Autodesk Inventor part; units mm, degrees
ref_plane "YZ Plane" through (0, 0, 0) normal (1, 0, 0) x (0, 1, 0)
ref_plane "XZ Plane" through (0, 0, 0) normal (0, 1, 0) x (-1, 0, 0)
ref_plane "XY Plane" through (0, 0, 0) normal (0, 0, 1) x (1, 0, 0)
sketch "Sketch1" plane through (0, 0, 0) normal (0, 0, 1) x (1, 0, 0)
  circle A0 centre (0, 0) radius 1.621
  dimension "d0" = 3.242
extrude "Extrusion1" add sketch "Sketch1" along normal blind 4.6
sketch "Sketch2" plane through (0, 0, 4.6) normal (0, 0, 1) x (1, 0, 0)
  circle A0 centre (0, 0) radius 2.5
  dimension "d3" = 5
extrude "Extrusion2" add sketch "Sketch2" along normal blind 3
sketch "Sketch3" plane through (0, 0, 7.6) normal (0, 0, 1) x (1, 0, 0)
  line L0 (0.866, 1.5) -> (1.7321, 0)
  line L1 (1.7321, 0) -> (0.866, -1.5)
  line L2 (0.866, -1.5) -> (-0.866, -1.5)
  line L3 (-0.866, -1.5) -> (-1.7321, 0)
  line L4 (-1.7321, 0) -> (-0.866, 1.5)
  line L5 (-0.866, 1.5) -> (0.866, 1.5)
  point P0 (0, 0)
  dimension "d14" = 3
extrude "Extrusion3" cut sketch "Sketch3" against normal blind 2
thread "Thread1"
properties part number "M4 sujecion"
Check sheet for the modelled part. Datum: model origin and axes. Units: mm. A direction names the side the tool comes from. Give positions to 0.01 mm unless a question says otherwise; leave off trailing zeros. Order: outer loops, then holes, each group sorted by start corner. A loop starts at its lowest first (then second) coordinate and runs counter-clockwise, first axis right, second up. Notation, with made-up numbers: M -28,-19 L 4,-19 A11 ccw 4,-1 Z; hole C -23,78.25 d1. An arc over 180 degrees is marked long. Answer as CSV lines item,"result". Start each with the question number.
Item 1: Cross-section at A-A on z = 6.25. Enter the section's corners in (x, y).
Item 2: Mould release check, pull along Y, two halves, no side actions. Record for faces 1 (the face through (-0.54, 2.44, 6.08)), 2 (the face through (0, 0, 0)), 3 (the face through (0, -1.5, 7)): +Y half, -Y half, draft (parallel to the pull), parting line (faces both ways), or undercut.
Item 3: Cross-section at B-B on x = 0. Enter the section's corners in (y, z), plus the area to 3 significant figures.
Item 4: Gauge pin test, flat ends, axial feed: P1, Ø1, axis at x = -1, z = 5, coming from the +Y side; P2, Ø1.5, axis at x = 0.5, y = 0, coming from the +Z side; P3, Ø3, axis at x = -1, z = 1, coming from the +Y side. Record the tip position at first contact, or that the pin passes through.
Item 5: Cross-section at C-C on y = 1.2. Enter the section's corners in (x, z).
Item 6: Cross-section at D-D on z = 2.5. Enter the section's corners in (x, y), plus the area to 4 significant figures.
Item 7: Tool access check on faces 4 (the face through (-1.305, 0.74, 6.614)), 5 (the face through (0.748, 1.438, 2.268)), 6 (the face through (0, -2, 7.6)). Record the directions out of +Z, -Z, +X, -X, +Y, -Y that give a thin tool (end or side, any length) a straight path to the whole face; none if there is none.
Item 8: Thickness scan on line 1 (Y direction, x = -2, z = 4.75); line 2 (Z direction, x = -1.3, y = -0.3); line 3 (Z direction, x = -1.8, y = 1.15). Record the ranges inside material, lowest first. Write a range as [from, to].
Established:
1,outline,"C 0,0 d5; hole M -1.73,0 L -0.87,-1.5 L 0.87,-1.5 L 1.73,0 L 0.87,1.5 L -0.87,1.5 Z"
2,face 1,"parting line"
2,face 2,"draft"
2,face 3,"undercut"
3,outline,"M -2.5,4.6 L -1.62,4.6 L -1.62,0 L 1.62,0 L 1.62,4.6 L 2.5,4.6 L 2.5,7.6 L 1.5,7.6 L 1.5,5.6 L -1.5,5.6 L -1.5,7.6 L -2.5,7.6 Z"
3,area,"23.9 mm^2"
4,P1,"stops at y = 2.45"
4,P2,"stops at z = 5.6"
4,P3,"stops at y = 1.62"
5,outline,"M -2.19,4.6 L -1.09,4.6 L -1.09,0 L 1.09,0 L 1.09,4.6 L 2.19,4.6 L 2.19,7.6 L 1.04,7.6 L 1.04,5.6 L -1.04,5.6 L -1.04,7.6 L -2.19,7.6 Z"
6,outline,"C 0,0 d3.24"
6,area,"8.255 mm^2"
7,face 4,"+Z"
7,face 5,"-Z"
7,face 6,"+Z, +X, -X, +Y, -Y"
8,line 1,"y = [-1.5, 1.5]"
8,line 2,"z = [0, 5.6]"
8,line 3,"z = [4.6, 7.6]"
